Geometry check sheet. Reference: the model listing, model coordinates, mm. A direction names the side the tool comes from. Give positions to 0.01 mm unless a question says otherwise; leave off trailing zeros. Loops run counter-clockwise (first coordinate to the right, second up) from the corner with the lowest first, then second, coordinate; pieces in that order, holes last. Notation, with made-up numbers: (56, -18) -> (97, -18) arc R23 ccw to (97, 20) -> close; hole circle Ø11 at (51.5, 1.25). An arc over 180 degrees is marked (long way). One line per item, written item: value. Start each with the question number.
(1) Gauge pin test, flat ends, axial feed: pin 1 Ø4 at (x, y) = (0, 11.5) entering from +Z; pin 2 Ø0.5 at (x, z) = (-2, 1.5) entering from -Y. Record the tip position at first contact, or that the pin passes through.
(2) Tool access check on faces 1 (the face through (-8.167, 9.86, 1.493)), 2 (the face through (-17.481, -0.657, 1.493)), 3 (the face through (-3.2, -2.1, 1.5)), 4 (the face through (-5, 7, 0)), 5 (the face through (7.49, -1.51, 1.49)). Record the directions out of +Z, -Z, +X, -X, +Y, -Y that give a thin tool (end or side, any length) a straight path to the whole face; none if there is none.
(3) Draft check along Y on faces 6 (the face through (9.91, -2.28, 0.59)), 7 (the face through (-3, -0.9, 1.5)), 8 (the face through (-1.567, 21.692, 1.087)). Enter one of: pulls with the +Y half, pulls with the -Y half, needs draft (parallel to the pull), parting line crosses it, or undercut.
(4) Scan lines: line 1 along Y through (x, z) = (-3, 1.75); line 2 along Y through (x, z) = (-6.75, 1.2); line 3 along Z through (x, y) = (-3, 12.5). Record each from-to range of solid material in increasing order. Write a range as from..to.
(5) Sectioned sample at A-A, the plane z = 0.5. Record the cut outline in (x, y).
from build123d import *

# Parameters (mm, degrees)
F2_DEPTH    = 1
F4_DEPTH    = 1
F5_T1_DEPTH = 13.9032439889
F5_T3_DEPTH = 12.9032439889
F6_R        = 4
F7_DEPTH    = 0.4
F10_R       = 0.2


# Not quite as in the source:
# - a fillet or chamfer that OpenCascade refuses, or shapes differently, is made with other operations: its cross-section is extruded or revolved along the edge and cut away or added


with BuildPart() as f2:
    # F0 (on Top) → F2 (new body)
    with BuildSketch(Plane.XY):
        Polygon((0, 20), (-16.1091689951, 0), (9.5716667723, 0), align=None)
    extrude(amount=F2_DEPTH)



with BuildPart() as f2b:
    # F1 (on face) → F2, piece 2 (new body)
    with BuildSketch(Plane.XY):
        with BuildLine():
            Line((-1.4357500158, 23), (-18.4455415549, 1.8818510201))
            ThreePointArc((-18.4455415549, 1.8818510201), (-18.8152319157, -1.295076627), (-16.1091689951, -3))
            Line((-16.1091689951, -3), (11.0074167882, -3))
            Line((11.0074167882, -3), (9.5716667723, 0))
            Line((9.5716667723, 0), (-16.1091689951, 0))
            Line((-16.1091689951, 0), (0, 20))
            Line((0, 20), (-1.4357500158, 23))
        make_face()
    extrude(amount=F2_DEPTH)


with BuildPart() as f2_1:
    add(f2.part)

    add(f2b.part)  # F4 merges F2b
    # F3 (on face) → F4 (join)
    with BuildSketch(Plane.XY.offset(1)):
        with BuildLine():
            Line((-18.8152319157, -1.295076627), (-16.1091689951, 0))
            Line((-16.1091689951, 0), (0, 20))
            Line((0, 20), (-1.4357500158, 23))
            Line((-1.4357500158, 23), (-18.4455415549, 1.8818510201))
            ThreePointArc((-18.4455415549, 1.8818510201), (-19.0890609751, 0.3467618604), (-18.8152319157, -1.295076627))
        make_face()
        with BuildLine():
            ThreePointArc((-14.928229743, 2.9009278658), (-15.771874459, 2.8100235579), (-15.8627787669, 3.6536682739))
            Line((-15.8627787669, 3.6536682739), (-3.3171052997, 19.2294853393))
            ThreePointArc((-3.3171052997, 19.2294853393), (-2.4734605837, 19.3203896472), (-2.3825562758, 18.4767449312))
            Line((-2.3825562758, 18.4767449312), (-14.928229743, 2.9009278658))
        make_face(mode=Mode.SUBTRACT)
        with BuildLine():
            Line((6.8908310049, -0.9), (-13.1091689951, -0.9))
            ThreePointArc((-13.1091689951, -0.9), (-13.7091689951, -1.5), (-13.1091689951, -2.1))
            Line((-13.1091689951, -2.1), (6.8908310049, -2.1))
            ThreePointArc((6.8908310049, -2.1), (7.4908310049, -1.5), (6.8908310049, -0.9))
        make_face()
    extrude(amount=F4_DEPTH)

    # F5: fillet of radius 1.5 on 2 edges, made by hand

    # F5_s2 → F5_t1 (cut)
    with BuildSketch(Plane.XY.offset(-5.9516219944)):
        with BuildLine():
            ThreePointArc((-0.4079522763, 20.8526480249), (-1.5876028064, 21.6950557014), (-2.9291700165, 21.1460352214))
            Line((-2.9291700165, 21.1460352214), (-2.9525337421, 21.1648537316))
            ThreePointArc((-2.9525337421, 21.1648537316), (-2.2057848022, 22.0918047567), (-1.4591137414, 23.0188185102))
            Line((-1.4591137414, 23.0188185102), (-1.4086893866, 23.0129507663))
            ThreePointArc((-1.4086893866, 23.0129507663), (-0.8948356179, 21.9392531941), (-0.3808916471, 20.8655987912))
            Line((-0.3808916471, 20.8655987912), (-0.4079522763, 20.8526480249))
        make_face()
    extrude(amount=F5_T1_DEPTH, mode=Mode.SUBTRACT)

    # F5_s4 → F5_t3 (cut)
    with BuildSketch(Plane.XY.offset(-5.9516219944)):
        with BuildLine():
            ThreePointArc((9.9797994528, -0.8525616865), (9.8958833281, -2.2996913111), (8.6267679925, -3.0001))
            Line((8.6267679925, -3.0001), (8.6267679925, -3.0301))
            ThreePointArc((8.6267679925, -3.0301), (9.8170923903, -3.03), (11.0074167882, -3.03))
            Line((11.0074167882, -3.03), (11.0344774174, -2.9870492337))
            ThreePointArc((11.0344774174, -2.9870492337), (10.5206236486, -1.9133516616), (10.006860082, -0.8396109202))
            Line((10.006860082, -0.8396109202), (9.9797994528, -0.8525616865))
        make_face()
    extrude(amount=F5_T3_DEPTH, mode=Mode.SUBTRACT)

    # F6 (on face) → F7 (join)
    with BuildSketch(Plane.XY.offset(1)):
        with Locations((0, 7.70957988)):
            Circle(F6_R)
    extrude(amount=F7_DEPTH)

    # F8: fillet of radius 6 on 1 edges, made by hand

    # F8_s1 → F8_t2 (revolve, cut)
    with BuildSketch(Plane.XZ.offset(-7.70957988)):
        with BuildLine():
            ThreePointArc((4, 1), (2.9413791922, 1.2991524815), (1.8459340771, 1.4))
            Line((1.8459340771, 1.4), (4, 1.4))
            Line((4, 1.4), (4, 1))
        make_face()
    revolve(axis=Axis((0, 7.70957988, 1.4), (0, 0, 1)), mode=Mode.SUBTRACT)

    # F9: union 

    # F10
    f10_edges = [f2_1.edges().sort_by_distance(p)[0] for p in [
        (4.785833, 10, 0),
        (-1.587603, 21.695056, 0),
        (-10.681885, 11.520656, 0),
        (-18.815232, -1.295077, 0),
        (-3.73254, -3, 0),
        (9.895883, -2.299691, 0),
    ]]
    fillet(f10_edges, radius=F10_R)


solid = f2_1.part
Calculated:
1. pin 1: stops at z = 1.4
1. pin 2: stops at y = -2.1
2. face 1: +Z
2. face 2: +Z, -Y
2. face 3: +Z, +X, -X, -Y
2. face 4: -Z, +X, -X, +Y, -Y
2. face 5: +Z, +X
3. face 6: parting line crosses it
3. face 7: undercut
3. face 8: pulls with the +Y half
4. line 1: y = -2.1..-0.9, 16.28..17.71, 19.43..21.06
4. line 2: y = -2.1..-0.9, 11.62..13.05, 14.97..16.4
4. line 3: z = 0..1
5. outline: (-18.45, 1.88) arc R3 ccw to (-16.11, -3) -> (8.64, -3) arc R1.5 ccw to (9.99, -0.87) -> (-0.42, 20.87) arc R1.5 ccw to (-2.92, 21.16) -> close
